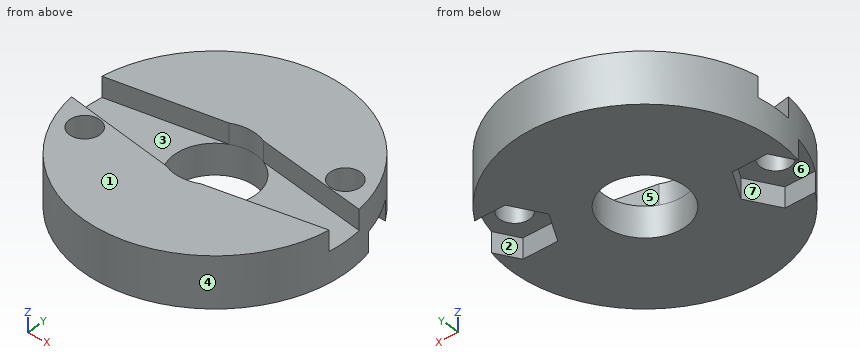
```python
from build123d import *

# Parameters (mm, degrees)
CYLINDER_R         = 13
CYLINDER_DEPTH     = 5
POCKET_DEPTH       = 2
SKETCH001_R        = 4
POCKET001_DEPTH    = 5.001
SKETCH002_R        = 1.5
POCKET002_DEPTH    = 5.001
POCKET003_DEPTH    = 2
POLARPATTERN_COUNT = 2


with BuildPart() as part:
    # Cylinder → Cylinder (new body)
    with BuildSketch(Plane.XY.offset(1)):
        Circle(CYLINDER_R)
    extrude(amount=CYLINDER_DEPTH)

    # Sketch → Pocket (cut)
    with BuildSketch(Plane.XY.offset(6)):
        with BuildLine():
            ThreePointArc((1.723508, 3.609643), (0, 4), (-1.723508, 3.609643))
            Line((-14.42367, 1.54169), (-1.723508, 3.609643))
            ThreePointArc((-14.42367, 1.54169), (-15.682586, 0.068213), (-14.437528, -1.416991))
            Line((-14.437528, -1.416991), (-1.723508, -3.609643))
            ThreePointArc((-1.723508, -3.609643), (0, -4), (1.723508, -3.609643))
            Line((1.723508, -3.609643), (14.437528, -1.416991))
            ThreePointArc((14.437528, -1.416991), (15.682586, 0.068213), (14.42367, 1.54169))
            Line((1.723508, 3.609643), (14.42367, 1.54169))
        make_face()
    extrude(amount=-POCKET_DEPTH, mode=Mode.SUBTRACT)

    # Sketch001 → Pocket001 (cut, through all)
    with BuildSketch(Plane.XY.offset(6)):
        Circle(SKETCH001_R)
    extrude(amount=-POCKET001_DEPTH, mode=Mode.SUBTRACT)

    # Sketch002 → Pocket002 (cut, through all)
    with BuildSketch(Plane.XY.offset(6)):
        with Locations((-9.617032, -3.94996)):
            Circle(SKETCH002_R)
        with Locations((9.617032, 3.94996)):
            Circle(SKETCH002_R)
    extrude(amount=-POCKET002_DEPTH, mode=Mode.SUBTRACT)

    # Sketch003 → Pocket003 (cut)
    with BuildSketch(Plane(origin=(0, 0, 1), x_dir=(1, 0, 0), z_dir=(0, 0, -1))):
        Polygon((-11.354812, 7.074793), (-7.854812, 7.074793), (-6.104812, 4.043704), (-7.854812, 1.012615), (-11.354812, 1.012615), (-13.104812, 4.043704), align=None)
    pocket003 = extrude(amount=-POCKET003_DEPTH, mode=Mode.SUBTRACT)

    # PolarPattern: Pocket003 ×2 about axis
    polarpattern_axis = Axis((0, 0, 1), (0, 0, -1))
    for i in range(1, POLARPATTERN_COUNT):
        add(pocket003.rotate(polarpattern_axis, i * 360 / POLARPATTERN_COUNT), mode=Mode.SUBTRACT)


solid = part.part
```
Verification items for the finished model (mm, model axes). Face numbers are marked on the shaded views. A direction names the side the tool comes from. Give positions to 0.01 mm unless a question says otherwise; leave off trailing zeros. Loops run counter-clockwise (first coordinate to the right, second up) from the corner with the lowest first, then second, coordinate; pieces in that order, holes last. Notation, with made-up numbers: M 76.5,87 L 125.5,87 A22 cw 125.5,105 Z; hole C 15,4 d6. An arc over 180 degrees is marked long. Return JSON: item names as keys, results as strings.
1) Material ranges on L1, parallel to X at y = 3.5, z = 3.6; L2, parallel to X at y = 2.75, z = 1.4; L3, parallel to Y at x = -10, z = 5, recorded low to high. Write a range as [from, to].
Findings:
{"L1": "x = [-12.52, -1.94], [1.94, 8.19], [11.05, 12.52]", "L2": "x = [-12.71, -2.9], [2.9, 6.85], [12.36, 12.71]", "L3": "y = [-8.31, -5.4], [-2.5, -2.18], [2.26, 8.31]"}
2) Section check A-A, the plane y = 0. Enter the section's corners in (x, z), and give its area (3 significant figures).
Findings:
{"outline": "M -13,1 L -4,1 L -4,4 L -13,4 Z; M 4,1 L 13,1 L 13,4 L 4,4 Z", "area": "54.0 mm2"}
3) Mould release check, pull along Y, two halves, no side actions. Record for the marked faces 1, 2, 3 and 4: released by +Y, released by -Y, zero draft, split by the parting line, or undercut.
Findings:
{"face 1": "zero draft", "face 2": "released by +Y", "face 3": "undercut", "face 4": "split by the parting line"}
4) Section check C-C, the plane z = 5.5. Enter the section's corners in (x, y), and give its area (3 significant figures).
Findings:
{"outline": "M -12.89,-1.68 A13 ccw 12.89,-1.68 L 1.72,-3.61 A4 cw -1.72,-3.61 Z; M -12.88,1.79 L -1.72,3.61 A4 cw 1.72,3.61 L 12.88,1.79 A13 ccw Z; hole C -9.62,-3.95 d3; hole C 9.62,3.95 d3", "area": "370 mm2"}
5) Section check B-B, the plane x = 0. Enter the section's corners in (y, z).
Findings:
{"outline": "M -13,1 L -4,1 L -4,6 L -13,6 Z; M 4,1 L 13,1 L 13,6 L 4,6 Z"}
6) Section check D-D, the plane x = -10.25. Enter the section's corners in (y, z).
Findings:
{"outline": "M -8,1 L -7.07,1 L -7.07,3 L -5.31,3 L -5.31,6 L -8,6 Z; M -2.59,3 L -1.01,3 L -1.01,1 L 8,1 L 8,6 L 2.22,6 L 2.22,4 L -2.14,4 L -2.14,6 L -2.59,6 Z"}
7) Gauge pin test, flat ends, axial feed: P1, Ø1.6, axis at x = -10, z = 2, coming from the -Y side; P2, Ø1.8, axis at x = -11, y = -2.5, coming from the -Z side; P3, Ø2, axis at x = 10, z = 2, coming from the +Y side; P4, Ø7, axis at x = 0, y = 0, coming from the -Z side. Record the tip position at first contact, or that the pin passes through.
Findings:
{"P1": "stops at y = -9.18", "P2": "stops at z = 3", "P3": "stops at y = 9.38", "P4": "passes through"}
8) Tool access check on the marked faces 5, 6 and 7. Record the directions out of +Z, -Z, +X, -X, +Y, -Y that give a thin tool (end or side, any length) a straight path to the whole face; none if there is none.
Findings:
{"face 5": "+Z", "face 6": "-Z", "face 7": "-Z, -X"}
